For this review, take the finished solid that the model builds, in its own axes (mm). A direction names the side the tool comes from. Give positions to 0.01 mm unless a question says otherwise; leave off trailing zeros. Loops run counter-clockwise (first coordinate to the right, second up) from the corner with the lowest first, then second, coordinate; pieces in that order, holes last. Notation, with made-up numbers: (21.25, 46.5) -> (70.25, 46.5) arc R11 ccw to (70.25, 52.5) -> close; hole circle Ø11 at (-28, 14.25). An arc over 180 degrees is marked (long way). Answer as CSV lines item,"result". Start each with the question number.
Item 1: Add section C-C on z = 7.5. State how many separate pieces and enclosed holes the cut face has, plus the area to 3 significant figures.
Item 2: Add section A-A on x = -33. State the section outline as (y, z) points, plus the area to 3 significant figures.
Item 3: Add section B-B on y = -1. State the section outline as (x, z) points.
Item 4: Machinability: for faces 4 (the face through (-126.5, -1, 15)), 5 (the face through (128.94, -58.58, 15.21)), 6 (the face through (116.5, -1, 33)), which of the approach directions +Z, -Z, +X, -X, +Y, -Y give a long, thin tool a straight path to every point of the face, cutting with its end or side? Answer none if there is none.
Item 5: For L1, parallel to X at y = -50.95, z = 7.5; L2, parallel to Y at x = -25.5, z = 4; L3, parallel to X at y = -28, z = 9, list the stretches that pass through material, from the lowest coordinate up. Write a range as from..to.
Item 6: Clearance check with a flat-ended pin moving along its axis: P1, Ø3.5, axis at x = 121, z = 10.5, coming from the -Y side. State where the tip first meets the part, or that it passes through.
Item 7: The part is to be moulded in two halves that separate along Z. For faces 1 (the face through (122.035, 46.584, 15.415)), 2 (the face through (-128.94, -58.58, 15.21)), 3 (the face through (-1, 47, 30)), say which applies: +Z half, -Z half, draft (parallel to the pull), parting line (faces both ways), or undercut.
```python
from build123d import *

# Parameters (mm, degrees)
SKETCH1_W             = 263
SKETCH1_H             = 122
SKETCH1_W_2           = 253
SKETCH1_H_2           = 112
BOSS_EXTRUDE1_DEPTH   = 30
SKETCH1_W_3           = 249
SKETCH1_H_3           = 108
SKETCH1_W_4           = 239
SKETCH1_H_4           = 98
BOSS_EXTRUDE1_2_DEPTH = 30
SKETCH2_W             = 263
SKETCH2_H             = 122
BOSS_EXTRUDE2_DEPTH   = 5
FILLET1_R             = 1.5
SKETCH3_R             = 17.5
CUT_EXTRUDE1_DEPTH    = 12
FILLET2_R             = 3.5
FILLET3_R             = 8.5
FILLET4_R             = 5
SKETCH4_R             = 2.35
CUT_EXTRUDE2_DEPTH    = 279
SKETCH5_W             = 233
SKETCH5_H             = 92
CUT_EXTRUDE3_DEPTH    = 10


with BuildPart() as part:
    # Sketch1 → Boss-Extrude1 (new body)
    with BuildSketch(Plane.XY):
        Rectangle(SKETCH1_W, SKETCH1_H)
        Rectangle(SKETCH1_W_2, SKETCH1_H_2, mode=Mode.SUBTRACT)
    extrude(amount=BOSS_EXTRUDE1_DEPTH)



with BuildPart() as body_2:
    # Sketch1 → Boss-Extrude1 2 (new body)
    with BuildSketch(Plane.XY):
        Rectangle(SKETCH1_W_3, SKETCH1_H_3)
        Rectangle(SKETCH1_W_4, SKETCH1_H_4, mode=Mode.SUBTRACT)
    extrude(amount=BOSS_EXTRUDE1_2_DEPTH)


with BuildPart() as part_1:
    add(part.part)

    add(body_2.part)  # Boss-Extrude2 merges body 2
    # Sketch2 → Boss-Extrude2 (add)
    with BuildSketch(Plane.XY.offset(30)):
        Rectangle(SKETCH2_W, SKETCH2_H)
    extrude(amount=BOSS_EXTRUDE2_DEPTH)

    # Fillet1
    fillet1_edges = [part_1.edges().sort_by_distance(p)[0] for p in [
        (-124.5, -54, 15),
        (124.5, -54, 15),
        (124.5, 54, 15),
        (-124.5, 54, 15),
    ]]
    fillet(fillet1_edges, radius=FILLET1_R)

    # Sketch3 → Cut-Extrude1 (cut)
    with BuildSketch(Plane(origin=(0, -61, 0), x_dir=(-1, 0, 0), z_dir=(0, -1, 0))):
        with Locations((105, -7.5)):
            Circle(SKETCH3_R)
        with Locations((-105, -7.5)):
            Circle(SKETCH3_R)
    extrude(amount=-CUT_EXTRUDE1_DEPTH, mode=Mode.SUBTRACT)

    # Fillet2
    fillet2_edges = [part_1.edges().sort_by_distance(p)[0] for p in [
        (126.5, 56, 15),
        (-126.5, 56, 15),
        (-126.5, -56, 15),
        (126.5, -56, 15),
    ]]
    fillet(fillet2_edges, radius=FILLET2_R)

    # Fillet3
    fillet3_edges = [part_1.edges().sort_by_distance(p)[0] for p in [
        (-131.5, -61, 17.5),
        (-131.5, 61, 17.5),
        (131.5, 61, 17.5),
        (131.5, -61, 17.5),
    ]]
    fillet(fillet3_edges, radius=FILLET3_R)

    # Fillet4
    fillet4_edges = [part_1.edges().sort_by_distance(p)[0] for p in [
        (0, -61, 35),
        (-131.5, 0, 35),
        (131.5, 0, 35),
        (0, 61, 35),
        (-129.01040764, 58.51040764, 35),
        (129.01040764, 58.51040764, 35),
        (129.01040764, -58.51040764, 35),
        (-129.01040764, -58.51040764, 35),
    ]]
    fillet(fillet4_edges, radius=FILLET4_R)

    # Sketch4 → Cut-Extrude2 (cut)
    with BuildSketch(Plane(origin=(131.5, 0, 0), x_dir=(0, 0, -1), z_dir=(1, 0, 0))):
        with Locations(Location((-17.5, -44.5, 0), (0, 0, 90))):
            Circle(SKETCH4_R)
        with Locations(Location((-17.5, 45.5, 0), (0, 0, 90))):
            Circle(SKETCH4_R)
    extrude(amount=-CUT_EXTRUDE2_DEPTH, mode=Mode.SUBTRACT)

    # Sketch5 → Cut-Extrude3 (cut)
    with BuildSketch(Plane.XY.offset(35)):
        Rectangle(SKETCH5_W, SKETCH5_H)
    extrude(amount=-CUT_EXTRUDE3_DEPTH, mode=Mode.SUBTRACT)


solid = part_1.part
```
Computed values:
1,separate pieces,"4"
1,enclosed holes,"0"
1,area,"6,470 mm²"
2,outline,"(-61, 0) -> (-56, 0) -> (-56, 30) -> (-54, 30) -> (-54, 0) -> (-49, 0) -> (-49, 30) -> (-46, 30) -> (-46, 35) -> (-56, 35) arc R5 ccw to (-61, 30) -> close; (46, 30) -> (49, 30) -> (49, 0) -> (54, 0) -> (54, 30) -> (56, 30) -> (56, 0) -> (61, 0) -> (61, 30) arc R5 ccw to (56, 35) -> (46, 35) -> close"
2,area,"739 mm²"
3,outline,"(-131.5, 0) -> (-126.5, 0) -> (-126.5, 30) -> (-124.5, 30) -> (-124.5, 0) -> (-119.5, 0) -> (-119.5, 30) -> (-116.5, 30) -> (-116.5, 35) -> (-126.5, 35) arc R5 ccw to (-131.5, 30) -> close; (116.5, 30) -> (119.5, 30) -> (119.5, 0) -> (124.5, 0) -> (124.5, 30) -> (126.5, 30) -> (126.5, 0) -> (131.5, 0) -> (131.5, 30) arc R5 ccw to (126.5, 35) -> (116.5, 35) -> close"
4,face 4,"-Z"
4,face 5,"+Z, -Z, +X, -Y"
4,face 6,"+Z, -Z"
5,L1,"-131.5..-126.5, -124.5..-122.5, -87.5..87.5, 122.5..124.5, 126.5..131.5"
5,L2,"-61..-56, -54..-49, 49..54, 56..61"
5,L3,"-131.5..-126.5, -124.5..-119.5, 119.5..124.5, 126.5..131.5"
6,P1,"y = -61"
7,face 1,"undercut"
7,face 2,"draft"
7,face 3,"-Z half"
